from build123d import *

# Parameters (mm, degrees)
SKETCH1_R          = 12.7
SKETCH3_R          = 107.95
CUT_EXTRUDE1_DEPTH = 1.5875


with BuildPart() as part:
    # Sketch1 → Revolve1 (revolve)
    with BuildSketch(Plane.XY):
        with Locations((101.6, 0)):
            Circle(SKETCH1_R)
    revolve(axis=Axis((0, 3.175, 0), (0, -1, 0)))

    # Sketch3 → Cut-Extrude1 (cut, symmetric)
    with BuildSketch(Plane(origin=(0, 0, 0), x_dir=(1, 0, 0), z_dir=(0, 1, 0))):
        Circle(SKETCH3_R)
        with BuildLine():
            ThreePointArc((27.757566502, -91.11575057), (67.351920908, -67.351920908), (91.11575057, -27.757566502))
            ThreePointArc((91.11575057, -27.757566502), (89.903527616, -21.822714376), (84.266922058, -19.60446461))
            ThreePointArc((84.266922058, -19.60446461), (40.804807613, -40.804807613), (19.60446461, -84.266922058))
            ThreePointArc((19.60446461, -84.266922058), (21.822714376, -89.903527616), (27.757566502, -91.11575057))
        make_face(mode=Mode.SUBTRACT)
        with BuildLine():
            ThreePointArc((-81.63869201, 23.668181818), (0, 38.1), (81.63869201, 23.668181818))
            ThreePointArc((81.63869201, 23.668181818), (88.283116885, 25.120584837), (89.802561211, 31.75))
            ThreePointArc((89.802561211, 31.75), (0, 95.25), (-89.802561211, 31.75))
            ThreePointArc((-89.802561211, 31.75), (-88.283116885, 25.120584837), (-81.63869201, 23.668181818))
        make_face(mode=Mode.SUBTRACT)
        with BuildLine():
            ThreePointArc((-84.266922058, -19.60446461), (-40.804807613, -40.804807613), (-19.60446461, -84.266922058))
            ThreePointArc((-19.60446461, -84.266922058), (-21.822714376, -89.903527616), (-27.757566502, -91.11575057))
            ThreePointArc((-27.757566502, -91.11575057), (-67.351920908, -67.351920908), (-91.11575057, -27.757566502))
            ThreePointArc((-91.11575057, -27.757566502), (-89.903527616, -21.822714376), (-84.266922058, -19.60446461))
        make_face(mode=Mode.SUBTRACT)
    extrude(amount=CUT_EXTRUDE1_DEPTH, both=True, mode=Mode.SUBTRACT)


solid = part.part
Source: CAD feature listing. Evaluate the final solid. Frame: model axes, mm. Give positions to 0.01 mm unless a question says otherwise; leave off trailing zeros. Write each loop counter-clockwise with the first axis right and the second up, starting at its lowest first coordinate (ties: lowest second). Pieces come first, ordered by that corner, then holes. Notation, with made-up numbers: M 40.25,88.5 L 66.25,88.5 A22 cw 66.25,119.5 Z; hole C -4,28.5 d9. An arc over 180 degrees is marked long. Return JSON: item names as keys, results as strings. Group by question number.
1) Cut plane A-A, the plane x = 75.5. Give the number of separate pieces and of enclosed holes in the cut face, then the cut area to 3 significant figures.
2) Ray query, L1, parallel to Z at x = 0, y = 0; L2, parallel to Z at x = 0, y = 1.25; L3, parallel to Z at x = -67.5, y = 9.5. Return the intervals inside material, ascending.
3) First-contact query: pin 1 Ø6 at (y, z) = (-5.5, 44.5) entering from +X; pin 2 Ø2 at (x, y) = (-26.5, 8.5) entering from -Z; pin 3 Ø8 at (y, z) = (-6, -45.5) entering from -X. Flat tips, straight axial feed; report the tip coordinate or a pass-through.
4) Cut plane C-C, the plane y = -5. Output: boundary loops of the cut face in (x, z).
Data:
{
 "1": {"separate pieces": "2", "enclosed holes": "2", "area": "1,420 mm²"},
 "2": {"L1": "z = -114.3 to -107.95, -95.25 to -88.9, 107.95 to 114.3", "L2": "z = -114.24 to -107.95, -95.25 to -88.96, 107.95 to 114.24", "L3": "z = -86.89 to -64.22, 64.22 to 86.89"},
 "3": {"pin 1": "stops at x = 105.67", "pin 2": "stops at z = -108.7", "pin 3": "stops at x = -105.62"},
 "4": {"outline": "C 0,0 d226.55; hole C 0,0 d179.85"}
}
